Source: three-view drawing plus pictorial views. Frame: mm from the lowest corner of the part. A direction names the side the tool comes from. Give positions to 0.01 mm unless a question says otherwise; leave off trailing zeros. Order: outer loops, then holes, each group sorted by start corner. A loop starts at its lowest first (then second) coordinate and runs counter-clockwise, first axis right, second up. Notation, with made-up numbers: (63.5, 60.5) -> (71.5, 60.5) arc R13 ccw to (71.5, 84.5) -> close; hole circle Ø7 at (70.25, -13). An arc over 180 degrees is marked (long way). Answer in a Markdown table with one row per item.
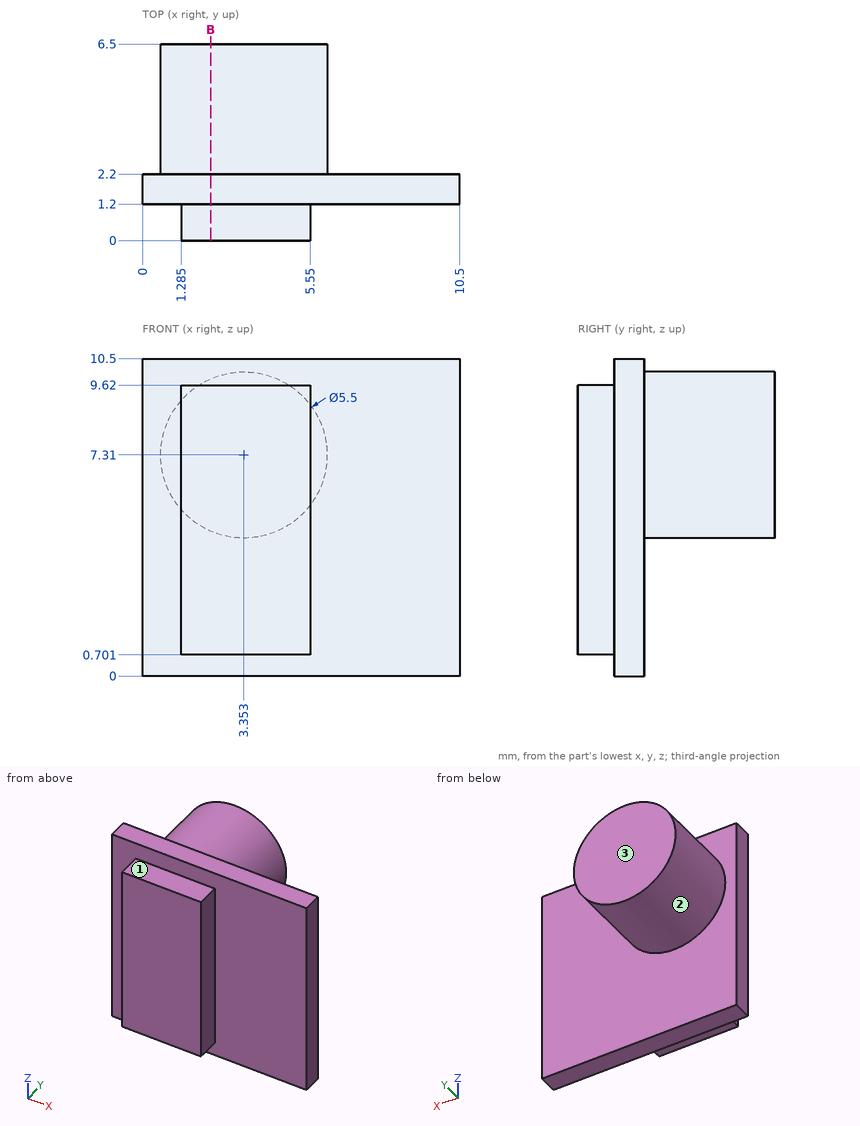
(1) Section query B-B (x = 2.25). Return the cut outline in (y, z).
A:
| item | result |
|---|---|
| outline | (0, 0.7) -> (1.2, 0.7) -> (1.2, 0) -> (2.2, 0) -> (2.2, 4.79) -> (6.5, 4.79) -> (6.5, 9.83) -> (2.2, 9.83) -> (2.2, 10.5) -> (1.2, 10.5) -> (1.2, 9.62) -> (0, 9.62) -> close |
(2) Ray query, probe 1 along Y at (x, z) = (6.5, 2.75); probe 2 along Z at (x, y) = (3.5, 5) (1 decimal); probe 3 along Z at (x, y) = (5.25, 0.75). Return the intervals inside material, ascending.
A:
| item | result |
|---|---|
| probe 1 | y = 1.2 to 2.2 |
| probe 2 | z = 4.6 to 10.1 |
| probe 3 | z = 0.7 to 9.62 |
(3) First-contact query: pin 1 Ø1.3 at (x, y) = (3.5, 0.5) entering from -Z; pin 2 Ø0.6 at (y, z) = (0.5, 6) entering from -X (1 decimal). Flat tips, straight axial feed; report the tip coordinate or a pass-through.
A:
| item | result |
|---|---|
| pin 1 | stops at z = 0.7 |
| pin 2 | stops at x = 1.3 |
(4) Access query for the marked faces 1, 2 and 3. Directions: +Z, -Z, +X, -X, +Y, -Y. A direction counts if a zero-diameter tool reaches every point of the face in a straight line with its end or side. Return the directions, or none.
A:
| item | result |
|---|---|
| face 1 | +Z, +X, -X, -Y |
| face 2 | +Y |
| face 3 | +Z, -Z, +X, -X, +Y |
